from build123d import *

# Parameters (mm, degrees)
SKETCH1_W           = 4
SKETCH1_H           = 17
BOSS_EXTRUDE1_DEPTH = 6
SKETCH2_W           = 2.8
SKETCH2_H           = 6.5
SKETCH2_W_2         = 1.5
SKETCH2_H_2         = 2.75
CUT_EXTRUDE1_DEPTH  = 19.466185313
CUT_EXTRUDE2_DEPTH  = 19.466185313
SKETCH4_W           = 2
SKETCH4_H           = 2.75
BOSS_EXTRUDE2_DEPTH = 2
SKETCH5_W           = 1.2
SKETCH5_H           = 12
BOSS_EXTRUDE3_DEPTH = 2
SKETCH6_W           = 1.5
SKETCH6_H           = 1.5
SKETCH6_H_2         = 0.75
CUT_EXTRUDE3_DEPTH  = 2


with BuildPart() as part:
    # Sketch1 → Boss-Extrude1 (new body)
    with BuildSketch(Plane.XY):
        with Locations((2, 8.5)):
            Rectangle(SKETCH1_W, SKETCH1_H)
    extrude(amount=BOSS_EXTRUDE1_DEPTH)

    # Sketch2 → Cut-Extrude1 (cut, through all)
    with BuildSketch(Plane.XY.offset(6)):
        with Locations((2.6, 9.25)):
            Rectangle(SKETCH2_W, SKETCH2_H)
        with Locations((3.25, 3.875)):
            Rectangle(SKETCH2_W_2, SKETCH2_H_2)
    extrude(amount=-CUT_EXTRUDE1_DEPTH, mode=Mode.SUBTRACT)

    # Sketch3 → Cut-Extrude2 (cut, through all)
    with BuildSketch(Plane.ZY):
        Polygon((0, 15.25), (0.75, 14.25), (0.75, 15.25), (2, 15.25), (2, 1.75), (0.75, 1.75), (0.75, 2.75), (0, 1.75), align=None)
    extrude(amount=-CUT_EXTRUDE2_DEPTH, mode=Mode.SUBTRACT)

    # Sketch4 → Boss-Extrude2 (add)
    with BuildSketch(Plane(origin=(4, 0, 0), x_dir=(0, 0, -1), z_dir=(1, 0, 0))):
        with Locations((-5, 3.875)):
            Rectangle(SKETCH4_W, SKETCH4_H)
    extrude(amount=-BOSS_EXTRUDE2_DEPTH)

    # Sketch5 → Boss-Extrude3 (add)
    with BuildSketch(Plane.XY.offset(6)):
        with Locations((0.6, 8.5)):
            Rectangle(SKETCH5_W, SKETCH5_H)
    extrude(amount=BOSS_EXTRUDE3_DEPTH)

    # Sketch6 → Cut-Extrude3 (cut)
    with BuildSketch(Plane(origin=(0, 0, 2), x_dir=(-1, 0, 0), z_dir=(0, 0, -1))):
        with Locations((-3.25, 13.25)):
            Rectangle(SKETCH6_W, SKETCH6_H)
        with Locations((-3.25, 5.625)):
            Rectangle(SKETCH6_W, SKETCH6_H_2)
    extrude(amount=-CUT_EXTRUDE3_DEPTH, mode=Mode.SUBTRACT)


solid = part.part
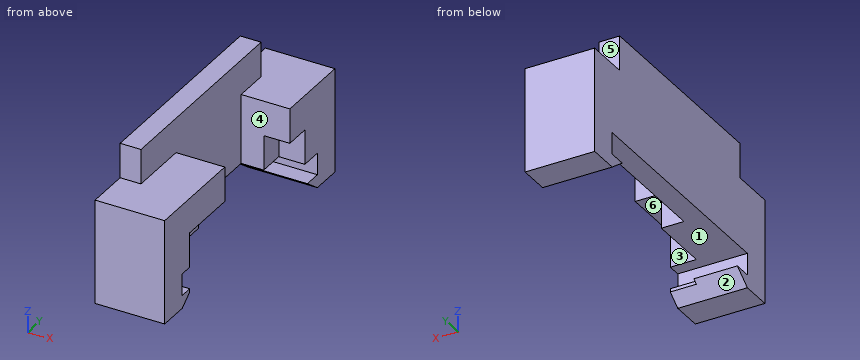
For this review, take the finished solid that the model builds, in its own axes (mm). Face numbers are marked on the shaded views. A direction names the side the tool comes from. Give positions to 0.01 mm unless a question says otherwise; leave off trailing zeros. Order: outer loops, then holes, each group sorted by start corner. A loop starts at its lowest first (then second) coordinate and runs counter-clockwise, first axis right, second up. Notation, with made-up numbers: (80.5, 65.5) - (92.5, 65.5) arc R25 ccw to (92.5, 93.5) - close; hole circle Ø5 at (20.25, -15). An arc over 180 degrees is marked (long way). Answer as a JSON object with one key per item and string values. Group by question number.
Item 1: Wall thickness on line 1 along Y through (x, z) = (2.1, 4); line 2 along Y through (x, z) = (3.75, 3.75); line 3 along Z through (x, y) = (3.3, 12.75): over which ranges is each line inside the solid? List them lowest first.
Item 2: Take a section at C-C on y = 3.5. Give the boundary of the cut face in (x, z).
Item 3: Machinability: for the marked faces 4, 5 and 6, which of the approach directions +Z, -Z, +X, -X, +Y, -Y give a long, thin tool a straight path to every point of the face, cutting with its end or side? Answer none if there is none.
Item 4: Draft analysis for pull direction Z (two halves, no side actions). For the marked faces 1, 2 and 3, state which applies: pulls with the +Z half, pulls with the -Z half, needs draft (parallel to the pull), parting line crosses it, or undercut.
Item 5: Clearance check with flat-ended pins moving along their axes: pin 1 Ø0.5 at (x, y) = (2.5, 2.5) entering from +Z; pin 2 Ø1.6 at (x, y) = (3.5, 4) entering from -Z; pin 3 Ø1.3 at (x, z) = (0.5, 7) entering from -Y. State where each tip first meets the part, or that it passes through.
Item 6: Take a section at D-D on z = 4.25. Give the boundary of the cut face in (x, y), and give its area (3 significant figures).
Item 7: Take a section at B-B on z = 1. Give the boundary of the cut face in (x, y).
Item 8: Take a section at A-A on x = 2.95. Give the boundary of the cut face in (y, z), and give its area (3 significant figures).
Reported:
{
 "1": {"line 1": "0 to 6, 12.5 to 17", "line 2": "0 to 2.5, 14 to 17", "line 3": "4 to 6"},
 "2": {"outline": "(0, 2) - (2.5, 2) - (2.5, 4) - (4, 4) - (4, 6) - (1.2, 6) - (1.2, 8) - (0, 8) - close"},
 "3": {"face 4": "+Z, -Z, +X", "face 5": "+Z, +X, -X, +Y", "face 6": "-Z, +X"},
 "4": {"face 1": "undercut", "face 2": "pulls with the -Z half", "face 3": "needs draft"},
 "5": {"pin 1": "z = 6", "pin 2": "z = 4", "pin 3": "y = 2.5"},
 "6": {"outline": "(0, 0) - (4, 0) - (4, 6) - (1.2, 6) - (1.2, 12.5) - (4, 12.5) - (4, 17) - (0, 17) - close", "area": "49.8 mm^2"},
 "7": {"outline": "(0, 0) - (4, 0) - (4, 1.75) - (0, 1.75) - close; (0, 15.25) - (4, 15.25) - (4, 17) - (0, 17) - close"},
 "8": {"outline": "(0, 0) - (1.75, 0) - (2.5, 0.56) - (2.5, 0.75) - (1.75, 0.75) - (1.75, 2) - (2.5, 2) - (2.5, 4) - (6, 4) - (6, 6) - (0, 6) - close; (12.5, 4) - (14, 4) - (14, 2) - (15.25, 2) - (15.25, 0.75) - (14.25, 0.75) - (15.25, 0) - (17, 0) - (17, 6) - (12.5, 6) - close", "area": "39.7 mm^2"}
}
